```python
from build123d import *

# Parameters (mm, degrees)
SKETCH1_W                 = 110
SKETCH1_H                 = 85
BASE_DEPTH                = 25
FILLET1_R                 = 5
SKETCH2_W                 = 96.5
SKETCH2_H                 = 73
BASKET_DEPTH              = 19
SKETCH3_W                 = 4
SKETCH3_H                 = 6
WIRE_CHANNEL_DEPTH        = 19
WIRE_CHANNEL_ROUNDING_R   = 1
SWITCH_CUT_OUT_REACH      = 106.283
SKETCH5_W                 = 17
SKETCH5_H                 = 15
SWITCH_CUT_OUT_ROUNDING_R = 3
SKETCH14_R                = 1.75
CORNER_HOLES_DEPTH        = 74.866433513
BOTTOM_NUT_CUT_OUT_DEPTH  = 3
SKETCH18_W                = 8.304257035
SKETCH18_H                = 5.473277891
PRINTING_TIE_DOWNS_DEPTH  = 0.5


with BuildPart() as part:
    # Sketch1 → Base (new body)
    with BuildSketch(Plane(origin=(0, 0, 0), x_dir=(1, 0, 0), z_dir=(0, 1, 0))):
        Rectangle(SKETCH1_W, SKETCH1_H)
    extrude(amount=BASE_DEPTH)

    # Fillet1
    fillet1_edges = [part.edges().sort_by_distance(p)[0] for p in [
        (55, 12.5, 42.5),
        (-55, 12.5, 42.5),
        (-55, 12.5, -42.5),
        (55, 12.5, -42.5),
    ]]
    fillet(fillet1_edges, radius=FILLET1_R)

    # Sketch2 → Basket (cut)
    with BuildSketch(Plane(origin=(0, 25, 0), x_dir=(1, 0, 0), z_dir=(0, 1, 0))):
        Rectangle(SKETCH2_W, SKETCH2_H)
    extrude(amount=-BASKET_DEPTH, mode=Mode.SUBTRACT)

    # Sketch3 → Wire Channel (cut)
    with BuildSketch(Plane(origin=(0, 25, 0), x_dir=(1, 0, 0), z_dir=(0, 1, 0))):
        with Locations((-15, -36.5)):
            Rectangle(SKETCH3_W, SKETCH3_H)
    extrude(amount=-WIRE_CHANNEL_DEPTH, mode=Mode.SUBTRACT)

    # Wire Channel Rounding
    wire_channel_rounding_edges = [part.edges().sort_by_distance(p)[0] for p in [
        (-17, 15.5, 39.5),
        (-13, 15.5, 39.5),
    ]]
    fillet(wire_channel_rounding_edges, radius=WIRE_CHANNEL_ROUNDING_R)

    # Sketch5 → Switch Cut-out (cut, up to next)
    with BuildSketch(Plane.XY.offset(42.5), mode=Mode.PRIVATE) as switch_cut_out_sk1:
        with Locations((-34.75, 17.5)):
            Rectangle(SKETCH5_W, SKETCH5_H)
    switch_cut_out_tool1 = extrude(switch_cut_out_sk1.sketch, amount=-SWITCH_CUT_OUT_REACH, mode=Mode.PRIVATE) & part.part
    add(switch_cut_out_tool1.solids().sort_by_distance((-34.75, 17.5, 42.5))[0], mode=Mode.SUBTRACT)

    # Switch Cut-out Rounding
    switch_cut_out_rounding_edges = [part.edges().sort_by_distance(p)[0] for p in [
        (-43.25, 17.5, 42.5),
        (-34.75, 10, 42.5),
        (-26.25, 17.5, 42.5),
    ]]
    fillet(switch_cut_out_rounding_edges, radius=SWITCH_CUT_OUT_ROUNDING_R)

    # Sketch14 → Corner Holes (cut, through all)
    with BuildSketch(Plane(origin=(0, 25, 0), x_dir=(1, 0, 0), z_dir=(0, 1, 0))):
        with Locations(Location((-50.892766953, 38.767766953, 0), (0, 0, 270))):
            Circle(SKETCH14_R)
        with Locations(Location((50.892766953, 38.767766953, 0), (0, 0, 270))):
            Circle(SKETCH14_R)
        with Locations(Location((50.892766953, -38.767766953, 0), (0, 0, 270))):
            Circle(SKETCH14_R)
        with Locations(Location((-50.892766953, -38.767766953, 0), (0, 0, 270))):
            Circle(SKETCH14_R)
    extrude(amount=-CORNER_HOLES_DEPTH, mode=Mode.SUBTRACT)

    # Sketch15 → Bottom Nut Cut-out (cut)
    with BuildSketch(Plane.XZ):
        Polygon((-50.64101323, 42.388469214), (-52.178282629, 43.416097239), (-55.727023172, 38.10739593), (-54.143831126, 37.15203238), (-51.13140477, 35.13829702), (-47.868872697, 36.746365575), (-47.630234881, 40.375835508), align=None)
        Polygon((50.595962101, 42.39294376), (52.091508492, 43.427758232), (55.676210978, 38.247033564), (54.180664587, 37.212219092), (51.189571805, 35.142590146), (47.901674171, 36.698138008), (47.604869319, 40.323314814), align=None)
        Polygon((54.167766953, -36.699113605), (55.742766953, -37.608440279), (52.313760602, -43.547653498), (50.738760602, -42.638326824), (47.463760602, -40.747504693), (47.463760602, -36.788029213), (50.892766953, -34.808291473), align=None)
        Polygon((-53.9527362, -36.801402743), (-55.569189191, -37.634817242), (-52.682156679, -43.23437466), (-51.065703688, -42.400960161), (-47.832797706, -40.734131163), (-47.65986097, -37.100937955), (-50.719830218, -35.134573745), align=None)
    extrude(amount=-BOTTOM_NUT_CUT_OUT_DEPTH, mode=Mode.SUBTRACT)

    # Sketch18 → Printing Tie-downs (add)
    with BuildSketch(Plane.XZ):
        Polygon((-50.728122477, 42.446699673), (-50.728122477, 50.804257035), (-45.254844585, 50.804257035), (-45.254844585, 42.5), align=None)
        Polygon((54.992489727, 37.773945836), (64.927443113, 37.773945836), (64.927443113, 32.300667944), (55, 32.300667944), align=None)
        Polygon((50.462105691, -42.478600037), (50.462105691, -51.181840402), (44.9888278, -51.181840402), (44.9888278, -42.5), align=None)
        with Locations((-59.152128518, -34.604714443)):
            Rectangle(SKETCH18_W, SKETCH18_H)
    extrude(amount=-PRINTING_TIE_DOWNS_DEPTH)


solid = part.part
```
Verification items for the finished model (mm, model axes). A direction names the side the tool comes from. Round coordinates to 2 decimals unless told otherwise and drop trailing zeros. Write each loop counter-clockwise with the first axis right and the second up, starting at its lowest first coordinate (ties: lowest second). Pieces come first, ordered by that corner, then holes.
1. Section check A-A on y = 8.5. Enter the section's corners in (x, z), plus the area to 3 significant figures.
2. Gauge pin test, flat ends, axial feed: P1, Ø6, axis at x = -59.5, z = -36, coming from the +Y side; P2, Ø10, axis at y = 3.5, z = -3, coming from the -X side; P3, Ø10, axis at x = -6.5, z = 4.5, coming from the +Y side. Record the tip position at first contact, or that the pin passes through.
3. Section check D-D on y = 18. Enter the section's corners in (x, z).
4. Scan lines: L1, parallel to Z at x = 46.5, y = 12.75; L2, parallel to X at y = 21, z = -35; L3, parallel to Z at x = 49.5, y = 13. Record each from-to range of solid material in increasing order.
5. Section check B-B on x = 13. Enter the section's corners in (y, z), plus the area to 3 significant figures.
6. Draft check along Z on faces 1 (the cylindrical face through (-53.57, 12.68, -41)), 2 (the flat face through (-49.17, 1.48, -36.13)), 3 (the flat face through (2, 0, 1)). Enter one of: +Z half, -Z half, draft (parallel to the pull), parting line (faces both ways), or undercut.
7. Section check C-C on z = -2. Enter the section's corners in (x, y), plus the area to 4 significant figures.
8. Access from +Z, -Z, +X, -X, +Y, -Y to the whole of each face (thin tool, end or side, straight path). Record for faces 4 (the flat face through (-43.25, 17, 38)), 5 (the flat face through (-48, 0.5, 47)), 6 (the flat face through (49.57, 1.48, 35.91)), 7 (the flat face through (-59, 0.5, -35)), 8 (the flat face through (-33, 9, 36.5)).
Answer:
1. outline: (-55, -37.5) arc R5 ccw to (-50, -42.5) - (50, -42.5) arc R5 ccw to (55, -37.5) - (55, 37.5) arc R5 ccw to (50, 42.5) - (-23.25, 42.5) arc R3 ccw to (-24.75, 42.1) - (-44.75, 42.1) arc R3 ccw to (-46.25, 42.5) - (-50, 42.5) arc R5 ccw to (-55, 37.5) - close; hole circle Ø3.5 at (-50.89, -38.77); hole circle Ø3.5 at (-50.89, 38.77); hole (-48.25, -36.5) - (48.25, -36.5) - (48.25, 36.5) - (-13, 36.5) - (-13, 38.5) arc R1 ccw to (-14, 39.5) - (-16, 39.5) arc R1 ccw to (-17, 38.5) - (-17, 36.5) - (-48.25, 36.5) - close; hole circle Ø3.5 at (50.89, -38.77); hole circle Ø3.5 at (50.89, 38.77)
1. area: 2,230 mm2
2. P1: stops at y = 0.5
2. P2: stops at x = -55
2. P3: stops at y = 6
3. outline: (-55, -37.5) arc R5 ccw to (-50, -42.5) - (50, -42.5) arc R5 ccw to (55, -37.5) - (55, 37.5) arc R5 ccw to (50, 42.5) - (-23.25, 42.5) arc R3 ccw to (-26.25, 39.5) - (-26.25, 36.5) - (-17, 36.5) - (-17, 38.5) arc R1 cw to (-16, 39.5) - (-14, 39.5) arc R1 cw to (-13, 38.5) - (-13, 36.5) - (48.25, 36.5) - (48.25, -36.5) - (-48.25, -36.5) - (-48.25, 36.5) - (-43.25, 36.5) - (-43.25, 39.5) arc R3 ccw to (-46.25, 42.5) - (-50, 42.5) arc R5 ccw to (-55, 37.5) - close; hole circle Ø3.5 at (-50.89, -38.77); hole circle Ø3.5 at (-50.89, 38.77); hole circle Ø3.5 at (50.89, -38.77); hole circle Ø3.5 at (50.89, 38.77)
4. L1: z = -42.5 to -36.5, 36.5 to 42.5
4. L2: x = -55 to -48.25, 48.25 to 55
4. L3: z = -42.5 to -39.83, -37.71 to 37.71, 39.83 to 42.5
5. outline: (0, -42.5) - (25, -42.5) - (25, -36.5) - (6, -36.5) - (6, 36.5) - (25, 36.5) - (25, 42.5) - (0, 42.5) - close
5. area: 738 mm2
6. face 1: -Z half
6. face 2: undercut
6. face 3: draft
7. outline: (-55, 0) - (55, 0) - (55, 25) - (48.25, 25) - (48.25, 6) - (-48.25, 6) - (-48.25, 25) - (-55, 25) - close
7. area: 916.5 mm2
8. face 4: +Z, +Y
8. face 5: +Z, +X, -X, +Y
8. face 6: -Y
8. face 7: +Z, -Z, -X, +Y
8. face 8: +Y
